The model under review builds one solid part; all positions refer to its coordinate system, in mm. A direction names the side the tool comes from. Round coordinates to 2 decimals unless told otherwise and drop trailing zeros. Loops run counter-clockwise (first coordinate to the right, second up) from the corner with the lowest first, then second, coordinate; pieces in that order, holes last. Notation, with made-up numbers: (2, 87) - (9, 87) arc R11 cw to (9, 101) - close; hole circle Ø11 at (1.25, -19). An arc over 180 degrees is marked (long way). Answer as CSV lines item,"result".
from build123d import *

# Parameters (mm, degrees)
SKETCH_W        = 40
SKETCH_H        = 24
PAD_DEPTH       = 3
SKETCH001_W     = 6
SKETCH001_H     = 24
PAD001_DEPTH    = 25
POCKET_DEPTH    = 6
POCKET001_DEPTH = 6
SKETCH005_R     = 1.5
POCKET002_DEPTH = 24.001
FILLET_R        = 3


with BuildPart() as part:
    # Sketch → Pad (new body)
    with BuildSketch(Plane.XY):
        Rectangle(SKETCH_W, SKETCH_H)
    extrude(amount=PAD_DEPTH)

    # Sketch001 (on Face6 of Pad) → Pad001 (join)
    with BuildSketch(Plane.XY.offset(3)):
        with Locations((-17, 0)):
            Rectangle(SKETCH001_W, SKETCH001_H)
        with Locations((17, 0)):
            Rectangle(SKETCH001_W, SKETCH001_H)
    extrude(amount=PAD001_DEPTH)

    # Sketch002 (on Face9 of Pad001) → Pocket (cut)
    with BuildSketch(Plane.YZ.offset(20)):
        with BuildLine():
            Line((-1.7, 28), (1.7, 28))
            Line((1.7, 28), (1.7, 13.999992))
            ThreePointArc((-1.7, 13.999989), (1e-06, 12.3), (1.7, 13.999992))
            Line((-1.7, 13.999989), (-1.7, 28))
        make_face()
    extrude(amount=-POCKET_DEPTH, mode=Mode.SUBTRACT)

    # Sketch004 (on Face12 of Pocket) → Pocket001 (cut)
    with BuildSketch(Plane(origin=(-20, 0, 0), x_dir=(0, -1, 0), z_dir=(-1, 0, 0))):
        with BuildLine():
            Line((-9.3, 28), (9.3, 28))
            Line((9.3, 28), (9.3, 14.000032))
            ThreePointArc((-9.3, 13.999973), (3e-05, 4.7), (9.3, 14.000032))
            Line((-9.3, 13.999973), (-9.3, 28))
        make_face()
    extrude(amount=-POCKET001_DEPTH, mode=Mode.SUBTRACT)

    # Sketch005 (on Face10 of Pocket001) → Pocket002 (cut, through all)
    with BuildSketch(Plane.XZ.offset(12)):
        with Locations((17, 21)):
            Circle(SKETCH005_R)
        with Locations((-17, 24)):
            Circle(SKETCH005_R)
    extrude(amount=-POCKET002_DEPTH, mode=Mode.SUBTRACT)

    # Fillet
    fillet_edges = [part.edges().sort_by_distance(p)[0] for p in [
        (-14, 0, 3),
        (14, 0, 3),
    ]]
    fillet(fillet_edges, radius=FILLET_R)


solid = part.part
1. Clearance check with flat-ended pins moving along their axes: pin 1 (2 mm diameter, centred on x = 11, y = 9.5, fed in from +Z); pin 2 (12 mm diameter, centred on y = -1, z = 23.5, fed in from -X); pin 3 (2.5 mm diameter, centred on x = 17, z = 21, fed in from -Y); pin 4 (6.5 mm diameter, centred on x = 3, y = -3.5, fed in from +Z). State where each tip first meets the part, or that it passes through.
Numbers:
pin 1,"stops at z = 3.17"
pin 2,"stops at x = 14"
pin 3,"passes through"
pin 4,"stops at z = 3"
2. Take a section at A-A (z = 24). State the section outline as (x, y) points, plus the area to 3 significant figures.
Numbers:
outline,"(-20, -12) - (-18.5, -12) - (-18.5, -9.3) - (-20, -9.3) - close; (-20, 9.3) - (-18.5, 9.3) - (-18.5, 12) - (-20, 12) - close; (-15.5, -12) - (-14, -12) - (-14, -9.3) - (-15.5, -9.3) - close; (-15.5, 9.3) - (-14, 9.3) - (-14, 12) - (-15.5, 12) - close; (14, -12) - (20, -12) - (20, -1.7) - (14, -1.7) - close; (14, 1.7) - (20, 1.7) - (20, 12) - (14, 12) - close"
area,"140 mm²"
3. Wall thickness on probe 1 along Y at (x, z) = (14.5, 25.5); probe 2 along Z at (x, y) = (17, -4.5); probe 3 along Z at (x, y) = (-17, -10.8): over which ranges is each line inside the solid? List them lowest first.
Numbers:
probe 1,"y = -12 to -1.7, 1.7 to 12"
probe 2,"z = 0 to 19.5, 22.5 to 28"
probe 3,"z = 0 to 22.5, 25.5 to 28"
4. Take a section at D-D (z = 21). State the section outline as (x, y) points.
Numbers:
outline,"(-20, -12) - (-14, -12) - (-14, -9.3) - (-20, -9.3) - close; (-20, 9.3) - (-14, 9.3) - (-14, 12) - (-20, 12) - close; (14, -12) - (15.5, -12) - (15.5, -1.7) - (14, -1.7) - close; (14, 1.7) - (15.5, 1.7) - (15.5, 12) - (14, 12) - close; (18.5, -12) - (20, -12) - (20, -1.7) - (18.5, -1.7) - close; (18.5, 1.7) - (20, 1.7) - (20, 12) - (18.5, 12) - close"
5. Draft analysis for pull direction Y (two halves, no side actions). For faces 1 (the face through (0, -12, 1)), 2 (the face through (17, 0, 12.3)), 3 (the face through (-17, -11, 28)), state which applies: +Y half, -Y half, draft (parallel to the pull), parting line (faces both ways), or undercut.
Numbers:
face 1,"-Y half"
face 2,"undercut"
face 3,"draft"
6. Take a section at B-B (x = 17). State the section outline as (y, z) points, plus the area to 3 significant figures.
Numbers:
outline,"(-12, 0) - (12, 0) - (12, 19.5) - (1.7, 19.5) - (1.7, 14) arc R1.7 cw to (-1.7, 14) - (-1.7, 19.5) - (-12, 19.5) - close; (-12, 22.5) - (-1.7, 22.5) - (-1.7, 28) - (-12, 28) - close; (1.7, 22.5) - (12, 22.5) - (12, 28) - (1.7, 28) - close"
area,"558 mm²"
7. Tool access review of faces 4 (the face through (20, 2, 14)), 5 (the face through (-17.042, 0.204, 4.702)), 6 (the face through (-13.14, -8.32, 3.9)): name each direction out of +Z, -Z, +X, -X, +Y, -Y from which nothing blocks a thin tool from reaching the whole face with its end or side.
Numbers:
face 4,"+Z, -Z, +X, +Y, -Y"
face 5,"+Z, -X"
face 6,"+Z, +Y, -Y"
8. Take a section at C-C (y = -10). State the section outline as (x, z) points.
Numbers:
outline,"(-20, 0) - (20, 0) - (20, 28) - (14, 28) - (14, 6) arc R3 cw to (11, 3) - (-11, 3) arc R3 cw to (-14, 6) - (-14, 28) - (-20, 28) - close; hole circle Ø3 at (-17, 24); hole circle Ø3 at (17, 21)"
